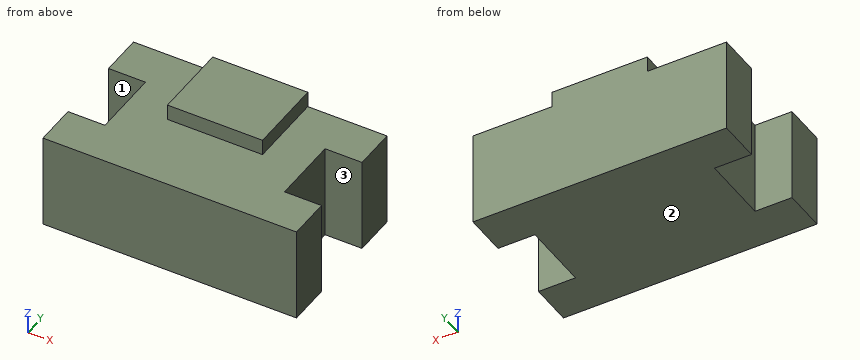
```python
from build123d import *

# Parameters (mm, degrees)
F0_W     = 152.4
F0_H     = 92.075
F1_DEPTH = 57.15
F2_W     = 57.15
F2_H     = 46.0375
F3_DEPTH = 9.525
F4_W     = 22.225
F4_H     = 41.275
F5_DEPTH = 57.15


with BuildPart() as f1:
    # F0 (on Top) → F1 (new body)
    with BuildSketch(Plane.XY):
        Rectangle(F0_W, F0_H)
    extrude(amount=F1_DEPTH)

    # F2 (on face) → F3 (join)
    with BuildSketch(Plane.XY.offset(57.15)):
        with Locations((0, 23.01875)):
            Rectangle(F2_W, F2_H)
    extrude(amount=F3_DEPTH)

    # F4 (on face) → F5 (cut)
    with BuildSketch(Plane.XY.offset(57.15)):
        with Locations((-65.0875, 0)):
            Rectangle(F4_W, F4_H)
        with Locations((65.0875, 0)):
            Rectangle(F4_W, F4_H)
    extrude(amount=-F5_DEPTH, mode=Mode.SUBTRACT)


solid = f1.part
```
Can you work these out from the model? Positions are in its coordinate system, mm. Face numbers are marked on the shaded views. A direction names the side the tool comes from. Coordinates: 2 decimals unless noted, no trailing zeros. Loops run counter-clockwise (first coordinate to the right, second up) from the corner with the lowest first, then second, coordinate; pieces in that order, holes last.
1) Imagine slicing it at A-A on x = 56.5. List the corners of the cut face in (y, z) for me.
2) Imagine slicing it at C-C on z = 18.5. List the corners of the cut face in (x, y) for me (1 decimal).
3) I need wall thicknesses on probe 1 along Y at (x, z) = (65.5, 16); probe 2 along Z at (x, y) = (-53.5, 10); probe 3 along X at (y, z) = (-8, 33.5) (3 decimals). Which ranges of each line are inside material? Lowest first, please.
4) Imagine slicing it at D-D on x = -31. List the corners of the cut face in (y, z) for me, plus the area to 3 significant figures.
5) For pin 1 (10.5 mm diameter, centred on y = 17, z = 61.5, fed in from +X) (3 decimals); pin 2 (3 mm diameter, centred on y = 19, z = 62.5, fed in from -X) (3 decimals); pin 3 (1.5 mm diameter, centred on x = -26.5, y = -32, fed in from -Z); pin 4 (5 mm diameter, centred on x = 14, z = 64, fed in from -Y), each with a flat end and sliding along its axis, tell me the tip position at first contact or that it passes through.
6) Imagine slicing it at B-B on y = 7.5. List the corners of the cut face in (x, z) for me (3 decimals), plus the area to 3 significant figures.
7) Which directions (+Z, -Z, +X, -X, +Y, -Y) give clear straight access to the entire face, cutting with the end or side of a thin tool? Please do the marked faces 1, 2 and 3.
Completed:
1. outline: (-46.04, 0) - (-20.64, 0) - (-20.64, 57.15) - (-46.04, 57.15) - close; (20.64, 0) - (46.04, 0) - (46.04, 57.15) - (20.64, 57.15) - close
2. outline: (-76.2, -46) - (76.2, -46) - (76.2, -20.6) - (54, -20.6) - (54, 20.6) - (76.2, 20.6) - (76.2, 46) - (-76.2, 46) - (-76.2, 20.6) - (-54, 20.6) - (-54, -20.6) - (-76.2, -20.6) - close
3. probe 1: y = -46.04 to -20.64, 20.64 to 46.04
3. probe 2: z = 0 to 57.15
3. probe 3: x = -53.975 to 53.975
4. outline: (-46.04, 0) - (46.04, 0) - (46.04, 57.15) - (-46.04, 57.15) - close
4. area: 5,260 mm2
5. pin 1: stops at x = 53.975
5. pin 2: stops at x = -28.575
5. pin 3: stops at z = 0
5. pin 4: stops at y = 0
6. outline: (-53.975, 0) - (53.975, 0) - (53.975, 57.15) - (28.575, 57.15) - (28.575, 66.675) - (-28.575, 66.675) - (-28.575, 57.15) - (-53.975, 57.15) - close
6. area: 6,710 mm2
7. face 1: +Z, -Z, -X
7. face 2: -Z, +X, -X, +Y, -Y
7. face 3: +Z, -Z, +X
